Geometry check sheet. Reference: the model listing, model coordinates, mm. A direction names the side the tool comes from. Round coordinates to 2 decimals unless told otherwise and drop trailing zeros. Order: outer loops, then holes, each group sorted by start corner. A loop starts at its lowest first (then second) coordinate and runs counter-clockwise, first axis right, second up. Notation, with made-up numbers: (71, 80) - (110, 80) arc R22 ccw to (110, 95) - close; hole circle Ø9 at (-22.5, 72). An arc over 180 degrees is marked (long way). Return JSON: item names as keys, results as strings. Group by question number.
Q1. Tool access check on faces 1 (the flat face through (2, 7, -47)), 2 (the cylindrical face through (8.191, 1.479, 8.072)), 3 (the flat face through (47, 7, 2)), 4 (the cylindrical face through (-57.56, 1.48, 58.76)). Record the directions out of +Z, -Z, +X, -X, +Y, -Y that give a thin tool (end or side, any length) a straight path to the whole face; none if there is none.
Q2. Draft check along X on faces 5 (the cylindrical face through (8.072, 1.479, -8.191)), 6 (the cylindrical face through (-17.83, -24.65, 80.3)), 7 (the flat face through (-48, 7, 2)). Enter one of: pulls with the +X half, pulls with the -X half, needs draft (parallel to the pull), parting line crosses it, or undercut.
Q3. Sectioned sample at C-C, the plane y = -46. Record the cut outline in (x, z), then the cut area to 3 significant figures.
Q4. Material ranges on line 1 along Z through (x, y) = (0, 0.8); line 2 along X through (y, z) = (2.5, -70.5); line 3 along Y through (x, z) = (68, 53), recorded low to high.
Q5. Gauge pin test, flat ends, axial feed: pin 1 Ø0.9 at (y, z) = (1, -14) entering from +X; pin 2 Ø2 at (y, z) = (-18.5, -18) entering from +X; pin 3 Ø1 at (x, y) = (2.5, 6.5) entering from +Z. Record the tip position at first contact, or that the pin passes through.
Autodesk Inventor part; units mm, degrees
ref_plane "YZ Plane" through (0, 0, 0) normal (1, 0, 0) x (0, 1, 0)
ref_plane "XZ Plane" through (0, 0, 0) normal (0, 1, 0) x (-1, 0, 0)
ref_plane "XY Plane" through (0, 0, 0) normal (0, 0, 1) x (1, 0, 0)
sketch "Szkic1" plane through (0, 0, 0) normal (0, 1, 0) x (-1, 0, 0)
  circle A0 centre (0, 0) radius 11.5
  circle A1 centre (0, 0) radius 3
  line L0 (6, 8) -> (-6, 8)
  line L1 (-6, 8) -> (-6, -8)
  line L2 (-6, -8) -> (6, -8)
  line L3 (6, -8) -> (6, 8)
  line L4 (6, 8) -> (-6, -8) construction
  line L5 (-6, 8) -> (6, -8) construction
  line L6 (0, 8) -> (6, 0)
  line L7 (6, 0) -> (0, -8)
  line L8 (0, -8) -> (-6, 0)
  line L9 (-6, 0) -> (0, 8)
  dimension "d0" = 23
  dimension "d1" = 6
  dimension "d2" = 16
  dimension "d3" = 12
extrude "Wyciągnięcie proste1" add sketch "Szkic1" along normal blind 3 contours A0 | L3 L6 L0 | L9 L1 L0 | L6 L7 L8 L9 | L3 L2 L7 | L8 L2 L1
sketch "Szkic2" plane through (0, 0, 0) normal (0, -1, 0) x (1, 0, 0)
  circle A0 centre (0, 0) radius 11.5
  line L0 (-11.5, 0) -> (-11.5, -3)
  line L1 (-11.5, -3) -> (-82.2, -3)
  line L2 (-82.2, -3) -> (-82.2, 3)
  line L3 (-82.2, 3) -> (-11.5, 3)
  line L4 (-11.5, 3) -> (-11.5, -3)
  line L5 (-11.5, 3) -> (-11.1018, 3)
  line L6 (-11.5, -3) -> (-11.1018, -3)
  circle A1 centre (0, 0) radius 3
  line L7 (3, -11.5) -> (3, -82.2)
  line L8 (-3, -82.2) -> (-3, -11.5)
  line L9 (3, -11.5) -> (3, -11.1018)
  line L10 (0, -11.5) -> (3, -11.5)
  line L11 (-3, -11.5) -> (-3, -11.1018)
  line L12 (-3, -11.5) -> (3, -11.5)
  line L13 (3, -82.2) -> (-3, -82.2)
  line L14 (11.5, 3) -> (82.2, 3)
  line L15 (82.2, -3) -> (11.5, -3)
  line L16 (11.5, 3) -> (11.1018, 3)
  line L17 (11.5, 0) -> (11.5, 3)
  line L18 (11.5, -3) -> (11.1018, -3)
  line L19 (11.5, -3) -> (11.5, 3)
  line L20 (82.2, 3) -> (82.2, -3)
  line L21 (-3, 11.5) -> (-3, 82.2)
  line L22 (3, 82.2) -> (3, 11.5)
  line L23 (-3, 11.5) -> (-3, 11.1018)
  line L24 (0, 11.5) -> (-3, 11.5)
  line L25 (3, 11.5) -> (3, 11.1018)
  line L26 (3, 11.5) -> (-3, 11.5)
  line L27 (-3, 82.2) -> (3, 82.2)
  circle A2 centre (0, 0) radius 82.2547
  circle A3 centre (0, 0) radius 89.2547
  point P0 (-11.5, 0)
  point P1 (0, -11.5)
  point P2 (11.5, 0)
  point P3 (0, 11.5)
  point P4 (11.5, 0)
  point P5 (11.5, 0)
  point P6 (11.5, 0)
  dimension "d15" = 70.7
  dimension "d17" = 6
  dimension "d18" = 3
  dimension "d21" = 360
  dimension "d23" = 7
extrude "Wyciągnięcie proste2" add sketch "Szkic2" against normal blind 3 contours L19 L18 A0 | A0 L16 L17 | L17 L14 L20 L15 L19 | A0 L26 L25 | L9 L10 A0 | A2 L20 | A0 L23 L24 | L24 L21 L27 L22 L26 | L12 L11 A0 | L10 L7 L13 L8 L12 | L27 A2 | A2 L13 | A0 L4 L5 | L6 L0 A0 | L3 L4 L0 L1 L2 | L2 A2 | A3
sketch "Szkic3" plane through (0, 3, 0) normal (0, 1, 0) x (1, 0, 0)
  line L0 (82.2, 3) -> (11.1018, 3)
  circle A0 centre (0, 0) radius 89.2547
  line L1 (0, 89.2547) -> (89.2547, 89.2547)
  line L2 (89.2547, 89.2547) -> (89.2547, 0)
  line L3 (89.2547, 0) -> (0, 0)
  line L4 (0, 0) -> (0, 89.2547)
  circle A1 centre (0, 0) radius 3
  line L5 (0, 0) -> (89.2547, 89.2547)
  circle A2 centre (60.6377, 60.6377) radius 3.5
  arc A3 (82.2, 3) -> (3, 82.2) centre (0, 0) ccw
  circle A4 centre (0, 85.7547) radius 3.5
  circle A5 centre (-60.6377, 60.6377) radius 3.5
  circle A6 centre (-85.7547, 0) radius 3.5
  circle A7 centre (-60.6377, -60.6377) radius 3.5
  circle A8 centre (0, -85.7547) radius 3.5
  circle A9 centre (60.6377, -60.6377) radius 3.5
  circle A10 centre (85.7547, 0) radius 3.5
  dimension "d42" = 360
hole "Otwór3" at (60.6377, 3, -60.6377) at (0, 3, -85.7547) at (-60.6377, 3, -60.6377) at (-85.7547, 3, 0) at (85.7547, 3, 0) at (-60.6377, 3, 60.6377) at (0, 3, 85.7547) at (60.6377, 3, 60.6377) direction (0, -1, 0) diameter 3.2 end through all
sketch "Szkic5" plane through (0, 3, 0) normal (0, 1, 0) x (1, 0, 0)
  line L0 (9.8995, -1.4142) -> (1.4142, -9.8995)
  line L1 (1.4142, -9.8995) -> (-9.8995, 1.4142)
  line L2 (-9.8995, 1.4142) -> (-1.4142, 9.8995)
  line L3 (-1.4142, 9.8995) -> (9.8995, -1.4142)
  arc A0 (3, -11.1018) -> (11.1018, -3) centre (0, 0) ccw
  arc A1 (-11.1018, -3) -> (-3, -11.1018) centre (0, 0) ccw
  line L4 (3, -11.1018) -> (-3, -11.1018)
  line L5 (5.6569, -5.6569) -> (4.2426, 4.2426)
  line L6 (4.2426, 4.2426) -> (-5.6569, 5.6569)
  line L7 (-5.6569, 5.6569) -> (-4.2426, -4.2426)
  line L8 (-4.2426, -4.2426) -> (5.6569, -5.6569)
  dimension "d57" = 45
  dimension "d58" = 12
  dimension "d59" = 16
  dimension "d60" = 6
  dimension "d61" = 8
hole "Otwór4" at (5.6569, 3, 5.6569) at (4.2426, 3, -4.2426) at (-5.6569, 3, -5.6569) at (-4.2426, 3, 4.2426) direction (0, -1, 0) diameter 2.1 end through all
sketch "Szkic6" plane through (0, 3, 0) normal (0, 1, 0) x (1, 0, 0)
  line L0 (-15.1018, 2) -> (-15.1018, 4)
  line L1 (-15.1018, 4) -> (-82.6018, 4)
  line L2 (-82.6018, 4) -> (-82.6018, 2)
  line L3 (-82.6018, 2) -> (-15.1018, 2)
  line L4 (-11.1018, 3) -> (-82.2, 3)
  line L5 (-4, -15.1018) -> (-4, -82.6018)
  line L6 (-2, -82.6018) -> (-2, -15.1018)
  line L7 (-4, -82.6018) -> (-2, -82.6018)
  line L8 (-2, -15.1018) -> (-4, -15.1018)
  line L9 (15.1018, -4) -> (82.6018, -4)
  line L10 (82.6018, -2) -> (15.1018, -2)
  line L11 (82.6018, -4) -> (82.6018, -2)
  line L12 (15.1018, -2) -> (15.1018, -4)
  line L13 (4, 15.1018) -> (4, 82.6018)
  line L14 (2, 82.6018) -> (2, 15.1018)
  line L15 (4, 82.6018) -> (2, 82.6018)
  line L16 (2, 15.1018) -> (4, 15.1018)
  line L17 (-82.6018, -2) -> (-82.6018, -4)
  line L18 (-82.6018, -4) -> (-15.1018, -4)
  line L19 (-15.1018, -4) -> (-15.1018, -2)
  line L20 (-15.1018, -2) -> (-82.6018, -2)
  line L21 (-82.2, -3) -> (-11.1018, -3)
  line L22 (4, -82.6018) -> (4, -15.1018)
  line L23 (2, -15.1018) -> (2, -82.6018)
  line L24 (2, -82.6018) -> (4, -82.6018)
  line L25 (4, -15.1018) -> (2, -15.1018)
  line L26 (82.6018, 4) -> (15.1018, 4)
  line L27 (15.1018, 2) -> (82.6018, 2)
  line L28 (82.6018, 2) -> (82.6018, 4)
  line L29 (15.1018, 4) -> (15.1018, 2)
  line L30 (-4, 82.6018) -> (-4, 15.1018)
  line L31 (-2, 15.1018) -> (-2, 82.6018)
  line L32 (-2, 82.6018) -> (-4, 82.6018)
  line L33 (-4, 15.1018) -> (-2, 15.1018)
  point P0 (0, 0)
  point P1 (-3, -82.2)
  point P2 (82.2, -3)
  point P3 (3, 82.2)
  dimension "d69" = 2
  dimension "d70" = 1
  dimension "d71" = 4
  dimension "d72" = 67.5
  dimension "d75" = 360
  dimension "d77" = 1
  dimension "d78" = 2
  dimension "d79" = 67.5
  dimension "d80" = 4
  dimension "d83" = 360
extrude "Wyciągnięcie proste4" add sketch "Szkic6" along normal blind 8 and the other way blind 3
sketch "Szkic7" plane through (-4, 0, 15.1018) normal (-1, 0, 0) x (0, 0, 1)
  line L0 (0, 11) -> (67.5, 11)
  line L1 (74.1529, 3) -> (-104.3565, 3)
  line L2 (67.5, 11) -> (63.5, 11)
  line L3 (63.5, 11) -> (63.5, 3)
  line L4 (63.5, 3) -> (67.5, 3)
  line L5 (67.5, 3) -> (67.5, 11)
  point P0 (-15.1018, 0)
  dimension "d89" = 4
extrude "Wyciągnięcie proste5" cut sketch "Szkic7" against normal blind 2
pattern_circular "Szyk kołowy1" count 4 over 360 about axis through (0, 0, 0) along (0, 1, 0) of "Wyciągnięcie proste5"
sketch "Szkic8" plane through (0, 0, 0) normal (0, -1, 0) x (1, 0, 0)
  circle A0 centre (0, 0) radius 79.2547
  circle A1 centre (0, 0) radius 3
  circle A2 centre (0, 0) radius 82.2547
  dimension "d95" = 164.5094
  dimension "d96" = 158.5094
extrude "Wyciągnięcie proste6" add sketch "Szkic8" along normal blind 50 contours A2
sketch "Szkic9" plane through (0, 3, 0) normal (0, 1, 0) x (1, 0, 0)
  circle A0 centre (0, 0) radius 3
  circle A1 centre (0, 0) radius 79.2547
  circle A2 centre (0, 0) radius 82.2547
  circle A3 centre (0, 0) radius 79.2547
  line L0 (-4, -82.1574) -> (-4, -79.1537)
  line L1 (-4, -82.1574) -> (-4, -79.1537)
  line L2 (-82.1574, 4) -> (-78.6018, 4)
  line L3 (-82.1574, 4) -> (-78.6018, 4)
  line L4 (-78.6018, 4) -> (-79.1537, 4)
  line L5 (4, 79.1537) -> (4, 15.1018)
  line L6 (4, 79.1537) -> (4, 82.1574)
  line L7 (79.1537, -4) -> (-82.1574, -4)
  line L8 (78.6018, -4) -> (78.6018, -2)
  arc A4 (-82.1574, -4) -> (-4, -82.1574) centre (0, 0) ccw
  line L9 (-6.4282, -82.0032) -> (-6.3234, -79.0015)
  point P0 (-6.3344, -79.0012)
  dimension "d100" = 3
  dimension "d101" = 2
equation "\"d77\" = d70"
equation "\"d78\" = d69"
equation "\"d79\" = d72"
equation "\"d80\" = d71"
properties part number "rama-silnik-dol-2"
Reply:
{
 "1": {"face 1": "+Z, -Z, +Y", "face 2": "+Y, -Y", "face 3": "+X, -X, +Y", "face 4": "+Y"},
 "2": {"face 5": "undercut", "face 6": "parting line crosses it", "face 7": "needs draft"},
 "3": {"outline": "circle Ø164.51 at (0, 0); hole circle Ø158.51 at (0, 0)", "area": "1,520 mm^2"},
 "4": {"line 1": "-89.25 to -87.35, -84.15 to -3, 3 to 84.15, 87.35 to 89.25", "line 2": "-54.74 to -42.37, -4 to 4, 42.37 to 54.74", "line 3": "0 to 3"},
 "5": {"pin 1": "x = 88.22", "pin 2": "x = 80.48", "pin 3": "z = 82.6"}
}
